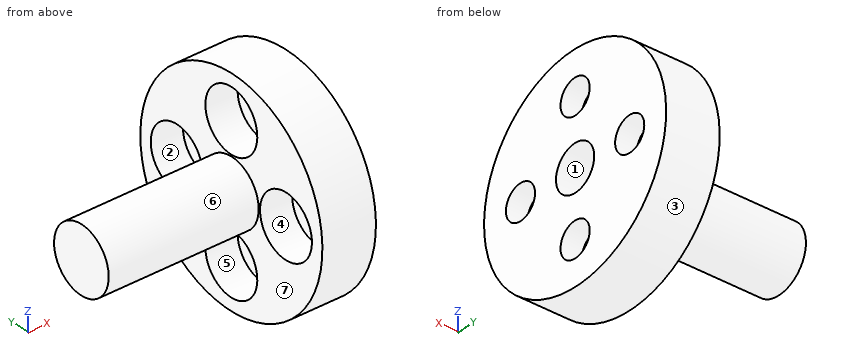
```python
from build123d import *

# Parameters (mm, degrees)
CUT_EXTRUDE1_DEPTH      = 24.685438565
CUT_EXTRUDE1_DEPTH_BACK = 24.685438565
SKETCH2_R               = 1.6
SKETCH3_R               = 2.85
CUT_EXTRUDE2_DEPTH      = 3


with BuildPart() as part:
    # Sketch1 → Revolve1 (revolve)
    with BuildSketch(Plane.XY, mode=Mode.PRIVATE) as revolve1_sk:
        Polygon((0, 2.1), (0, 10), (-5, 10), (-5, 3), (-19, 3), (-19, 0), (-13, 0), (-13, 2.1), align=None)
    revolve(revolve1_sk.sketch.rotate(Axis((-10, 0, 0), (1, 0, 0)), 90), axis=Axis((-10, 0, 0), (1, 0, 0)))

    # Sketch2 → Cut-Extrude1 (cut, two sides: drawn at the far end of the back side and taken through both)
    with BuildSketch(Plane(origin=(0, 0, 0), x_dir=(0, 0, -1), z_dir=(1, 0, 0)).offset(-CUT_EXTRUDE1_DEPTH_BACK)):
        with Locations((-6, 0)):
            Circle(SKETCH2_R)
        with Locations((6, 0)):
            Circle(SKETCH2_R)
        with Locations((0, 6)):
            Circle(SKETCH2_R)
        with Locations((0, -6)):
            Circle(SKETCH2_R)
    extrude(amount=CUT_EXTRUDE1_DEPTH + CUT_EXTRUDE1_DEPTH_BACK, mode=Mode.SUBTRACT)

    # Sketch3 → Cut-Extrude2 (cut)
    with BuildSketch(Plane(origin=(-5, 0, 0), x_dir=(0, 0, -1), z_dir=(1, 0, 0))):
        with Locations((-6, 0)):
            Circle(SKETCH3_R)
        with Locations((6, 0)):
            Circle(SKETCH3_R)
        with Locations((0, 6)):
            Circle(SKETCH3_R)
        with Locations((0, -6)):
            Circle(SKETCH3_R)
    extrude(amount=CUT_EXTRUDE2_DEPTH, mode=Mode.SUBTRACT)


solid = part.part
```
Design review of the part built by this model. Coordinates are the model's own, in mm. Face numbers are marked on the shaded views. A direction names the side the tool comes from. Give positions to 0.01 mm unless a question says otherwise; leave off trailing zeros. Write each loop counter-clockwise with the first axis right and the second up, starting at its lowest first coordinate (ties: lowest second). Pieces come first, ordered by that corner, then holes. Notation, with made-up numbers: (-25.75, -34.5) - (-14.75, -34.5) arc R14 cw to (-14.75, -12.5) - close; hole circle Ø11 at (-18.5, -9). An arc over 180 degrees is marked (long way). Return JSON: item names as keys, results as strings. Group by question number.
(1) We need section A-A, the plane y = 6. Give the boundary of the cut face in (x, z), then the cut area to 3 significant figures.
(2) Insertion check: pin 1 (4 mm diameter, centred on y = 6, z = 0, fed in from -X); pin 2 (3 mm diameter, centred on y = 1.5, z = -6, fed in from -X); pin 3 (1.5 mm diameter, centred on x = -14.5, y = 3.5, fed in from +Z). Each pin has a flat end and moves straight along its axis. Give the tip position at first contact, or say it passes through.
(3) We need section B-B, the plane z = 0. Give the boundary of the cut face in (x, y), then the cut area to 3 significant figures.
(4) We need section D-D, the plane y = -0.75. Give the boundary of the cut face in (x, z).
(5) Machinability: for the marked faces 1, 2 and 3, which of the approach directions +Z, -Z, +X, -X, +Y, -Y give a long, thin tool a straight path to every point of the face, cutting with its end or side? Answer none if there is none.
(6) We need section C-C, the plane x = -4.25. Give the boundary of the cut face in (y, z), then the cut area to 3 significant figures.
(7) Mouldability with a two-part tool opening along Y and no side actions: class the marked faces 4, 5, 6 and 7 as +Y half, -Y half, draft (parallel to the pull), parting line (faces both ways), or undercut.
(8) To check wall thickness, follow probe 1 along Y at (x, z) = (-3.3, 0); probe 2 along Y at (x, z) = (-0.35, 0); probe 3 along X at (y, z) = (-3.25, 7.25). State the ranges of each line that lie inside material, in increasing order.
Reported:
{
 "1": {"outline": "(-5, -8) - (0, -8) - (0, -1.6) - (-2, -1.6) - (-2, -2.85) - (-5, -2.85) - close; (-5, 2.85) - (-2, 2.85) - (-2, 1.6) - (0, 1.6) - (0, 8) - (-5, 8) - close", "area": "56.5 mm2"},
 "2": {"pin 1": "stops at x = -2", "pin 2": "stops at x = -5", "pin 3": "stops at z = 1.2"},
 "3": {"outline": "(-19, -3) - (-5, -3) - (-5, -3.15) - (-2, -3.15) - (-2, -4.4) - (0, -4.4) - (0, -2.1) - (-13, -2.1) - (-13, 2.1) - (0, 2.1) - (0, 4.4) - (-2, 4.4) - (-2, 3.15) - (-5, 3.15) - (-5, 3) - (-19, 3) - close; (-5, -10) - (0, -10) - (0, -7.6) - (-2, -7.6) - (-2, -8.85) - (-5, -8.85) - close; (-5, 8.85) - (-2, 8.85) - (-2, 7.6) - (0, 7.6) - (0, 10) - (-5, 10) - close", "area": "82.4 mm2"},
 "4": {"outline": "(-19, -2.9) - (-5, -2.9) - (-5, -3.25) - (-2, -3.25) - (-2, -4.59) - (0, -4.59) - (0, -1.96) - (-13, -1.96) - (-13, 1.96) - (0, 1.96) - (0, 4.59) - (-2, 4.59) - (-2, 3.25) - (-5, 3.25) - (-5, 2.9) - (-19, 2.9) - close; (-5, -9.97) - (0, -9.97) - (0, -7.41) - (-2, -7.41) - (-2, -8.75) - (-5, -8.75) - close; (-5, 8.75) - (-2, 8.75) - (-2, 7.41) - (0, 7.41) - (0, 9.97) - (-5, 9.97) - close"},
 "5": {"face 1": "+X", "face 2": "-X", "face 3": "+X, -X"},
 "6": {"outline": "circle Ø20 at (0, 0); hole circle Ø5.7 at (-6, 0); hole circle Ø5.7 at (0, -6); hole circle Ø5.7 at (0, 6); hole circle Ø4.2 at (0, 0); hole circle Ø5.7 at (6, 0)", "area": "198 mm2"},
 "7": {"face 4": "undercut", "face 5": "undercut", "face 6": "parting line", "face 7": "draft"},
 "8": {"probe 1": "y = -10 to -8.85, -3.15 to -2.1, 2.1 to 3.15, 8.85 to 10", "probe 2": "y = -10 to -7.6, -4.4 to -2.1, 2.1 to 4.4, 7.6 to 10", "probe 3": "x = -5 to 0"}
}
